Can you work these out from the model? Positions are in its coordinate system, mm. A direction names the side the tool comes from. Round coordinates to 2 decimals unless told otherwise and drop trailing zeros. Write each loop counter-clockwise with the first axis right and the second up, starting at its lowest first coordinate (ties: lowest second). Pieces come first, ordered by that corner, then holes.
Q1. For faces 1 (the flat face through (1.2, 0.7, -0.8)), 2 (the flat face through (1.2, -1.2, 0)), 3 (the cylindrical face through (-1.67, -0.53, -6.64)), which set-ups out of +Z, -Z, +X, -X, +Y, -Y let a thin tool reach every point of the face, with its end or its side?
Q2. We'd pull the mould along X, two halves only. Please class faces 4 (the flat face through (1.2, -0.7, -0.8)), 5 (the cylindrical face through (-2.278, -1.746, -1.728)), 6 (the flat face through (-1.2, -0.7, -0.8)), 7 (the flat face through (0, -2, -3.505)): +X half, -X half, draft (parallel to the pull), parting line (faces both ways), or undercut.
Q3. Please list where these lines run through material, in increasing order: line 1 along Z through (x, y) = (-2.3, -0.25); line 2 along Z through (x, y) = (-0.15, 1.1); line 3 along X through (y, z) = (0.2, -1).
Q4. I'm going to push flat-ended pins straight in: pin 1 Ø3 at (x, z) = (-1.5, -4.5) entering from +Y; pin 2 Ø0.8 at (x, y) = (0.5, -0.5) entering from +Z. Where does each tip first touch, or does it pass through?
Q5. If we section it at B-B (x = 0): Please give me the cut outline in (y, z), plus the area to 3 significant figures.
Q6. If we section it at A-A (z = -0.75): Please give me the cut outline in (x, y), plus the area to 3 significant figures.
Q7. If we section it at C-C (y = 0.5): Please give me the cut outline in (x, z).
Q8. If we section it at D-D (z = -2.75): Please give me the cut outline in (x, y), plus the area to 3 significant figures.
Autodesk Inventor part; units mm, degrees
ref_plane "YZ Plane" through (0, 0, 0) normal (1, 0, 0) x (0, 1, 0)
ref_plane "XZ Plane" through (0, 0, 0) normal (0, 1, 0) x (-1, 0, 0)
ref_plane "XY Plane" through (0, 0, 0) normal (0, 0, 1) x (1, 0, 0)
sketch "Sketch1" plane through (0, 0, 0) normal (0, 0, 1) x (1, 0, 0)
  circle A0 centre (0, 0) radius 2.8702
  dimension "head_dia" = 5.7404
extrude "Extrusion1" add sketch "Sketch1" against normal blind 3.5052
sketch "Sketch2" plane through (0, 0, -3.5052) normal (0, 0, -1) x (-1, 0, 0)
  circle A0 centre (0, 0) radius 1.7526
  dimension "body_dia" = 3.5052
extrude "Extrusion2" add sketch "Sketch2" along normal blind 6.35
sketch "Sketch3" plane through (0, 0, 0) normal (0, 0, 1) x (1, 0, 0)
  line L0 (1.604, 0) -> (0.802, -1.3891)
  line L1 (0.802, -1.3891) -> (-0.802, -1.3891)
  line L2 (-0.802, -1.3891) -> (-1.604, 0)
  line L3 (-1.604, 0) -> (-0.802, 1.3891)
  line L4 (-0.802, 1.3891) -> (0.802, 1.3891)
  line L5 (0.802, 1.3891) -> (1.604, 0)
  point P0 (0, 0)
  point P1 (0, 0)
  dimension "allen" = 2.7781
extrude "Extrusion3" cut sketch "Sketch3" against normal blind 1.6256
properties part number "shcs-6-0250"
A:
1. face 1: +Z
1. face 2: +Z, +X, -X, +Y, -Y
1. face 3: -Z
2. face 4: undercut
2. face 5: parting line
2. face 6: undercut
2. face 7: draft
3. line 1: z = -3.51 to 0
3. line 2: z = -9.86 to -1.63
3. line 3: x = -2.86 to -1.49, 1.49 to 2.86
4. pin 1: stops at y = 2.85
4. pin 2: stops at z = -1.63
5. outline: (-2.87, -3.51) - (-1.75, -3.51) - (-1.75, -9.86) - (1.75, -9.86) - (1.75, -3.51) - (2.87, -3.51) - (2.87, 0) - (1.39, 0) - (1.39, -1.63) - (-1.39, -1.63) - (-1.39, 0) - (-2.87, 0) - close
5. area: 37.9 mm2
6. outline: circle Ø5.74 at (0, 0); hole (-1.6, 0) - (-0.8, -1.39) - (0.8, -1.39) - (1.6, 0) - (0.8, 1.39) - (-0.8, 1.39) - close
6. area: 19.2 mm2
7. outline: (-2.83, -3.51) - (-1.68, -3.51) - (-1.68, -9.86) - (1.68, -9.86) - (1.68, -3.51) - (2.83, -3.51) - (2.83, 0) - (1.32, 0) - (1.32, -1.63) - (-1.32, -1.63) - (-1.32, 0) - (-2.83, 0) - close
8. outline: circle Ø5.74 at (0, 0)
8. area: 25.9 mm2
